Work out the finished part from the listing and answer in its coordinate system (mm). A direction names the side the tool comes from. Give positions to 0.01 mm unless a question says otherwise; leave off trailing zeros. Write each loop counter-clockwise with the first axis right and the second up, starting at its lowest first coordinate (ties: lowest second). Pieces come first, ordered by that corner, then holes. Notation, with made-up numbers: (61.25, 45.5) - (109.25, 45.5) arc R21 ccw to (109.25, 75.5) - close; hole circle Ø1 at (-8, -0.5). An arc over 180 degrees is marked (long way). Write item = value, one per line.
from build123d import *

# Parameters (mm, degrees)
SALIENTE_EXTRUIR1_DEPTH = 5
SALIENTE_EXTRUIR3_DEPTH = 19.374886
CROQUIS3_R              = 3.999935673
CORTAR_EXTRUIR2_DEPTH   = 45
SALIENTE_EXTRUIR4_DEPTH = 85.3
SALIENTE_EXTRUIR5_DEPTH = 15
SALIENTE_EXTRUIR6_DEPTH = 5
CHAFL_N1_SIZE           = 10


with BuildPart() as part:
    # Croquis1 → Saliente-Extruir1 (new body)
    with BuildSketch(Plane.XY):
        with BuildLine():
            Line((-10.200205365, -11.5), (-10.200205365, -4.721731506))
            ThreePointArc((-10.200205365, -4.721731506), (-11.240059515, 0), (-10.200205365, 4.721731506))
            Line((-10.200205365, 4.721731506), (-10.200205365, 21.15))
            Line((-10.200205365, 21.15), (-29.575095614, 21.15))
            Line((-29.575095614, 21.15), (-29.575095614, -26.15))
            Line((-29.575095614, -26.15), (-21.15, -26.15))
            Line((-21.15, -26.15), (21.175474863, -26.15))
            Line((21.175474863, -26.15), (21.15, -11.5))
            Line((21.15, -11.5), (21.124259996, 21.15))
            Line((21.124259996, 21.15), (11.5, 21.15))
            Line((11.5, 21.15), (11.5, -11.5))
            Line((11.5, -11.5), (-10.200205365, -11.5))
        make_face()
    extrude(amount=SALIENTE_EXTRUIR1_DEPTH)

    # Croquis2 → Saliente-Extruir3 (add)
    with BuildSketch(Plane.ZY.offset(29.575095614)):
        Polygon((5, 21.15), (28, 21.15), (28, -5.85), (5, -26.15), align=None)
    extrude(amount=-SALIENTE_EXTRUIR3_DEPTH)

    # Croquis3 → Cortar-Extruir2 (cut)
    with BuildSketch(Plane(origin=(0, 21.15, 0), x_dir=(1, 0, 0), z_dir=(0, 1, 0))):
        with Locations(Location((-17, -19.013114366, 0), (0, 0, 270))):
            Circle(CROQUIS3_R)
    extrude(amount=-CORTAR_EXTRUIR2_DEPTH, mode=Mode.SUBTRACT)

    # Croquis4 → Saliente-Extruir4 (add)
    with BuildSketch(Plane(origin=(0, 0, 0), x_dir=(-1, 0, 0), z_dir=(0, 0, -1))):
        Polygon((-21.175474863, -26.15), (29.575095614, -26.15), (29.575095614, 21.15), (21.575095614, 21.15), (21.575095614, -21.731968458), (-21.168633339, -21.731968458), align=None)
    extrude(amount=SALIENTE_EXTRUIR4_DEPTH)

    # Croquis5 → Saliente-Extruir5 (add)
    with BuildSketch(Plane(origin=(0, 0, -85.3), x_dir=(-1, 0, 0), z_dir=(0, 0, -1))):
        Polygon((-21.168633339, -21.731968458), (-21.102228651, 21.15), (29.575095614, 21.15), (29.575095614, -26.15), (-21.175474863, -26.15), align=None)
    extrude(amount=-SALIENTE_EXTRUIR5_DEPTH)

    # Croquis7 → Saliente-Extruir6 (add)
    with BuildSketch(Plane(origin=(21.134929711, 0.032728405, 0), x_dir=(0, 0, -1), z_dir=(0.9999988010052605, 0.0015485438455565383, 0))):
        Polygon((70.3, -21.764722958), (70.3, -6.93985202), (55.3, -21.764722958), align=None)
    extrude(amount=-SALIENTE_EXTRUIR6_DEPTH)

    # Chaflán1
    chafl_n1_edges = [part.edges().sort_by_distance(p)[0] for p in [
        (-29.575095614, 7.65, 28),
    ]]
    chamfer(chafl_n1_edges, length=CHAFL_N1_SIZE)


solid = part.part
1. Find section C-C, the plane z = 21. Give the vertices of the cut face in (x, y).
Solution:
outline = (-26.58, -12.03) - (-20.47, -12.03) - (-20.47, 21.15) - (-26.58, 21.15) - close; (-13.53, -12.03) - (-10.2, -12.03) - (-10.2, 21.15) - (-13.53, 21.15) - close
2. Given pin 1 (4 mm diameter, centred on x = 1.5, z = 3.5, fed in from +Y); pin 2 (1.5 mm diameter, centred on y = -9.5, z = 3, fed in from +X); pin 3 (10.5 mm diameter, centred on x = -17, z = 19.01, fed in from -Y), each flat-ended and moving along its own axis, determine where each tip first touches the part or whether it passes through.
Solution:
pin_1 = -11.5
pin_2 = 21.15
pin_3 = -18.42
3. Straight lines are drawn through the part: line 1 (Z direction, x = -17, y = 4); line 2 (Z direction, x = 5, y = -18.5); line 3 (X direction, y = 16.5, z = 13). For each, find the intervals that lie inside material, in ascending order.
Solution:
line_1 = -85.3 to -70.3, 0 to 15.01, 23.01 to 28
line_2 = -85.3 to -70.3, 0 to 5
line_3 = -29.58 to -10.2
4. Find section A-A, the plane x = 7.5. Give the vertices of the cut face in (y, z), then the cut area to 3 significant figures.
Solution:
outline = (-26.15, -85.3) - (21.15, -85.3) - (21.15, -70.3) - (-21.73, -70.3) - (-21.73, 0) - (-11.5, 0) - (-11.5, 5) - (-26.15, 5) - close
area = 1,090 mm^2
5. A tool of negligible diameter and unlimited length cuts with its end or side. For faces 4 (the flat face through (-1, -21.732, -35)), 5 (the cylindrical face through (-11.24, -0.07, 2.46)), 6 (the flat face through (-10.2, 3, 17)), 7 (the flat face through (-10.2, 13, 2)), from which of +Z, -Z, +X, -X, +Y, -Y can it reach the whole face along a straight path? Write none if from no direction.
Solution:
face_4 = +Y
face_5 = none
face_6 = +Z, +X, +Y, -Y
face_7 = +Z, +Y
6. Find section D-D, the plane x = -17. Give the vertices of the cut face in (y, z).
Solution:
outline = (-26.15, -85.3) - (21.15, -85.3) - (21.15, -70.3) - (-21.73, -70.3) - (-21.73, 0) - (21.15, 0) - (21.15, 15.01) - (-17.31, 15.01) - (-26.15, 5) - close; (-10.25, 23.01) - (21.15, 23.01) - (21.15, 28) - (-5.85, 28) - close
7. Find section B-B, the plane y = 3.5. Give the vertices of the cut face in (x, z).
Solution:
outline = (-29.58, -85.3) - (21.13, -85.3) - (21.13, -70.3) - (-21.58, -70.3) - (-21.58, 0) - (-10.68, 0) - (-10.68, 5) - (-10.2, 5) - (-10.2, 28) - (-19.58, 28) - (-29.58, 18) - close; (11.5, 0) - (21.14, 0) - (21.14, 5) - (11.5, 5) - close; hole circle Ø8 at (-17, 19.01)
8. For a pull along Z with two mould halves and no side action, classify faces 1 (the flat face through (-24.645, 7.468, 22.93)), 2 (the flat face through (-1, -14, 0)), 3 (the flat face through (-29.575, -3, -33)) as pulls with the +Z half, pulls with the -Z half, needs draft (parallel to the pull), parting line crosses it, or undercut.
Solution:
face_1 = pulls with the +Z half
face_2 = undercut
face_3 = needs draft
